from build123d import *

# Parameters (mm, degrees)
BOSS_EXTRU_1_DEPTH           = 6
ESQUISSE2_R                  = 5.5
ESQUISSE2_R_2                = 1.35
ESQUISSE2_R_3                = 2
ENL_V_MAT_EXTRU_1_DEPTH      = 1
ENL_V_MAT_EXTRU_1_DEPTH_BACK = 7


with BuildPart() as part:
    # Esquisse1 → Boss.-Extru.1 (new body)
    with BuildSketch(Plane.XY):
        with BuildLine():
            Line((12, 0), (8, 38))
            ThreePointArc((8, 38), (0, 46), (-8, 38))
            Line((-8, 38), (-12, 0))
            ThreePointArc((-12, 0), (0, -12), (12, 0))
        make_face()
    extrude(amount=BOSS_EXTRU_1_DEPTH)

    # Esquisse2 → Enlèv. mat.-Extru.1 (cut, two sides)
    with BuildSketch(Plane.XY.offset(6)) as enl_v_mat_extru_1_sk:
        Circle(ESQUISSE2_R)
        with Locations((8, 0)):
            Circle(ESQUISSE2_R_2)
        with Locations((0, -8)):
            Circle(ESQUISSE2_R_2)
        with Locations((-8, 0)):
            Circle(ESQUISSE2_R_2)
        with Locations((0, 8)):
            Circle(ESQUISSE2_R_2)
        with Locations((0, 38)):
            Circle(ESQUISSE2_R_3)
    extrude(amount=ENL_V_MAT_EXTRU_1_DEPTH, mode=Mode.SUBTRACT)
    extrude(enl_v_mat_extru_1_sk.sketch, amount=-ENL_V_MAT_EXTRU_1_DEPTH_BACK, mode=Mode.SUBTRACT)


solid = part.part
CAD build for the part. Positions are in the model's coordinates, mm. Coordinates: 2 decimals unless noted, no trailing zeros. Order: outer loops, then holes, each group sorted by start corner. A loop starts at its lowest first (then second) coordinate and runs counter-clockwise, first axis right, second up.
Item 1: Band-saw the part on C-C on y = -3. List the corners of the cut face in (x, z).
Check sheet entries:
outline: (-11.62, 0) - (-4.61, 0) - (-4.61, 6) - (-11.62, 6) - close; (4.61, 0) - (11.62, 0) - (11.62, 6) - (4.61, 6) - close
Item 2: Band-saw the part on D-D on x = 10.5. List the corners of the cut face in (y, z), plus the area to 3 significant figures.
Check sheet entries:
outline: (-5.81, 0) - (14.25, 0) - (14.25, 6) - (-5.81, 6) - close
area: 120 mm2
Item 3: Drill centre lines: L1, parallel to Y at x = 0, z = 3.3; L2, parallel to Y at x = 0.5, z = 0.3; L3, parallel to Y at x = 3, z = 2.75. Where is each one in solid material? Low to high.
Check sheet entries:
L1: y = -12 to -9.35, -6.65 to -5.5, 5.5 to 6.65, 9.35 to 36, 40 to 46
L2: y = -11.99 to -9.25, -6.75 to -5.48, 5.48 to 6.75, 9.25 to 36.06, 39.94 to 45.98
L3: y = -11.62 to -4.61, 4.61 to 45.42
Item 4: Two-plate mould, pull along X, no slides. Class faces 1 (the face through (0, 46, 3)), 2 (the face through (0, 36, 3)), 3 (the face through (0, 17, 6)): +X half, -X half, draft (parallel to the pull), parting line (faces both ways), or undercut.
Check sheet entries:
face 1: parting line
face 2: undercut
face 3: draft
Item 5: Band-saw the part on B-B on z = 5.05. List the corners of the cut face in (x, y).
Check sheet entries:
outline: (-12, 0) arc R12 ccw to (12, 0) - (8, 38) arc R8 ccw to (-8, 38) - close; hole circle Ø2.7 at (-8, 0); hole circle Ø11 at (0, 0); hole circle Ø4 at (0, 38); hole circle Ø2.7 at (0, -8); hole circle Ø2.7 at (0, 8); hole circle Ø2.7 at (8, 0)
Item 6: Band-saw the part on A-A on y = 39. List the corners of the cut face in (x, z), plus the area to 3 significant figures.
Check sheet entries:
outline: (-7.94, 0) - (-1.73, 0) - (-1.73, 6) - (-7.94, 6) - close; (1.73, 0) - (7.94, 0) - (7.94, 6) - (1.73, 6) - close
area: 74.5 mm2
Item 7: Pin check, flat tips, straight feed: pin 1 Ø1.5 at (x, z) = (8.5, 2.5) entering from -Y; pin 2 Ø3 at (x, z) = (-3, 2) entering from +Y; pin 3 Ø3 at (y, z) = (22, 2) entering from -X. Stop position of each tip, or through.
Check sheet entries:
pin 1: stops at y = -9.16
pin 2: stops at y = 45.86
pin 3: stops at x = -9.84
